Geometry check sheet. Reference: drawing and pictorial views, mm from the part's lowest x, y, z. A direction names the side the tool comes from. Coordinates: 2 decimals unless noted, no trailing zeros. Write each loop counter-clockwise with the first axis right and the second up, starting at its lowest first coordinate (ties: lowest second). Pieces come first, ordered by that corner, then holes. Notation, with made-up numbers: (35, 62) -> (61, 62) arc R9 ccw to (61, 75) -> close; hole circle Ø11 at (5, 4). An arc over 180 degrees is marked (long way). Use a Markdown table: item, result.
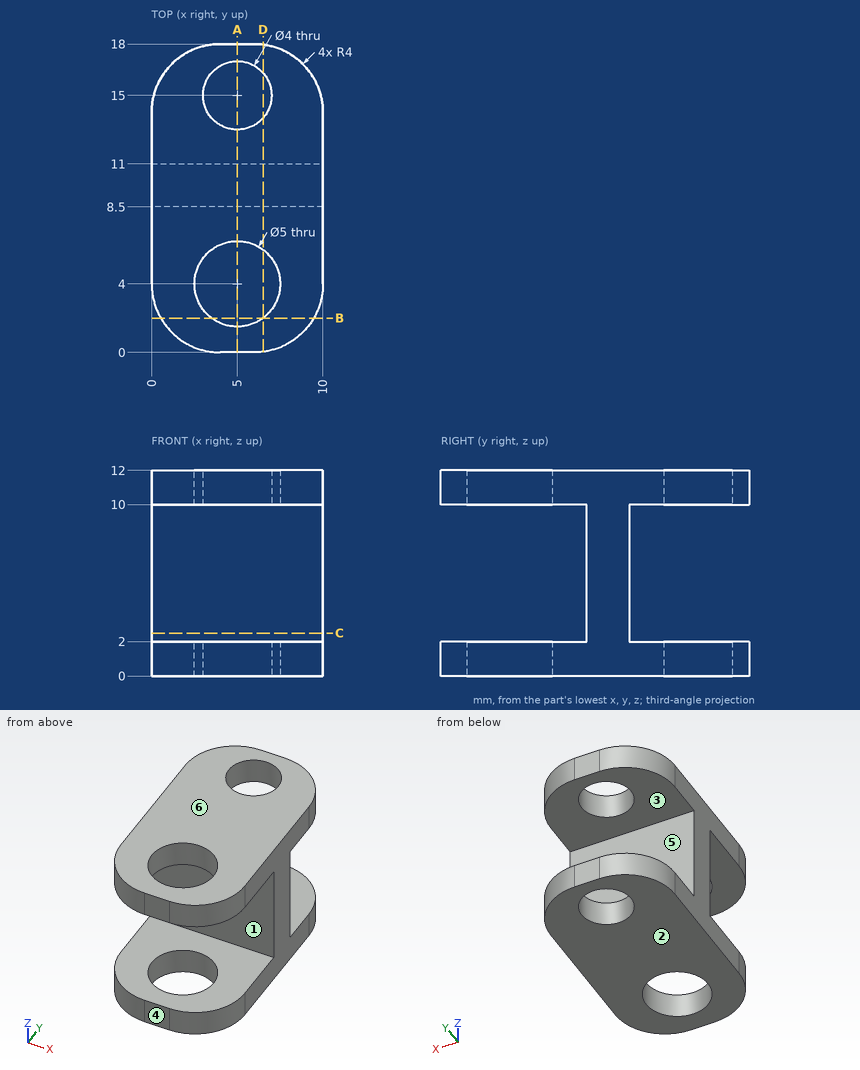
Item 1: Depth check by flat-ended pin: P1, Ø4.5, axis at x = 5, y = 4, coming from the -Z side; P2, Ø4, axis at x = 3, z = 7, coming from the -Y side. Enter the tip coordinate at first touch or a pass-through.
Answer block:
| item | result |
|---|---|
| P1 | passes through |
| P2 | stops at y = 8.5 |
Item 2: Section check A-A on x = 5. Record the boundary of the cut face in (y, z), then the cut area to 3 significant figures.
Answer block:
| item | result |
|---|---|
| outline | (0, 0) -> (1.5, 0) -> (1.5, 2) -> (0, 2) -> close; (0, 10) -> (1.5, 10) -> (1.5, 12) -> (0, 12) -> close; (6.5, 0) -> (13, 0) -> (13, 2) -> (11, 2) -> (11, 10) -> (13, 10) -> (13, 12) -> (6.5, 12) -> (6.5, 10) -> (8.5, 10) -> (8.5, 2) -> (6.5, 2) -> close; (17, 0) -> (18, 0) -> (18, 2) -> (17, 2) -> close; (17, 10) -> (18, 10) -> (18, 12) -> (17, 12) -> close |
| area | 56.0 mm^2 |
Item 3: Section check D-D on x = 6.5. Record the boundary of the cut face in (y, z).
Answer block:
| item | result |
|---|---|
| outline | (0.03, 0) -> (2, 0) -> (2, 2) -> (0.03, 2) -> close; (0.03, 10) -> (2, 10) -> (2, 12) -> (0.03, 12) -> close; (6, 0) -> (13.68, 0) -> (13.68, 2) -> (11, 2) -> (11, 10) -> (13.68, 10) -> (13.68, 12) -> (6, 12) -> (6, 10) -> (8.5, 10) -> (8.5, 2) -> (6, 2) -> close; (16.32, 0) -> (17.97, 0) -> (17.97, 2) -> (16.32, 2) -> close; (16.32, 10) -> (17.97, 10) -> (17.97, 12) -> (16.32, 12) -> close |
Item 4: Tool access check on the marked faces 1, 2 and 3. Record the directions out of +Z, -Z, +X, -X, +Y, -Y that give a thin tool (end or side, any length) a straight path to the whole face; none if there is none.
Answer block:
| item | result |
|---|---|
| face 1 | +X, -X, -Y |
| face 2 | -Z, +X, -X, +Y, -Y |
| face 3 | +X, -X, +Y |
Item 5: Section check C-C on z = 2.5. Record the boundary of the cut face in (x, y).
Answer block:
| item | result |
|---|---|
| outline | (0, 8.5) -> (10, 8.5) -> (10, 11) -> (0, 11) -> close |
Item 6: Thickness scan on L1, parallel to Y at x = 5, z = 1; L2, parallel to Z at x = 6.25, y = 12.75; L3, parallel to Y at x = 2, z = 2.5. Record the ranges inside material, lowest first. Write a range as [from, to].
Answer block:
| item | result |
|---|---|
| L1 | y = [0, 1.5], [6.5, 13], [17, 18] |
| L2 | z = [0, 2], [10, 12] |
| L3 | y = [8.5, 11] |
Item 7: Mould release check, pull along Z, two halves, no side actions. Record for the marked faces 4, 5 and 6: +Z half, -Z half, draft (parallel to the pull), parting line (faces both ways), or undercut.
Answer block:
| item | result |
|---|---|
| face 4 | draft |
| face 5 | undercut |
| face 6 | +Z half |
Item 8: Section check B-B on y = 2. Record the boundary of the cut face in (x, z).
Answer block:
| item | result |
|---|---|
| outline | (0.54, 0) -> (3.5, 0) -> (3.5, 2) -> (0.54, 2) -> close; (0.54, 10) -> (3.5, 10) -> (3.5, 12) -> (0.54, 12) -> close; (6.5, 0) -> (9.46, 0) -> (9.46, 2) -> (6.5, 2) -> close; (6.5, 10) -> (9.46, 10) -> (9.46, 12) -> (6.5, 12) -> close |
